Can you work these out from the drawing? Everything is in mm from the part's minimum corner. A direction names the side the tool comes from. Round coordinates to 2 decimals unless told otherwise and drop trailing zeros. Loops run counter-clockwise (first coordinate to the right, second up) from the corner with the lowest first, then second, coordinate; pieces in that order, holes last. Notation, with made-up numbers: (29, 57.25) -> (85, 57.25) arc R18 ccw to (85, 64.25) -> close; hole circle Ø6 at (69, -32). An arc over 180 degrees is marked (long way). One line per item, written item: value.
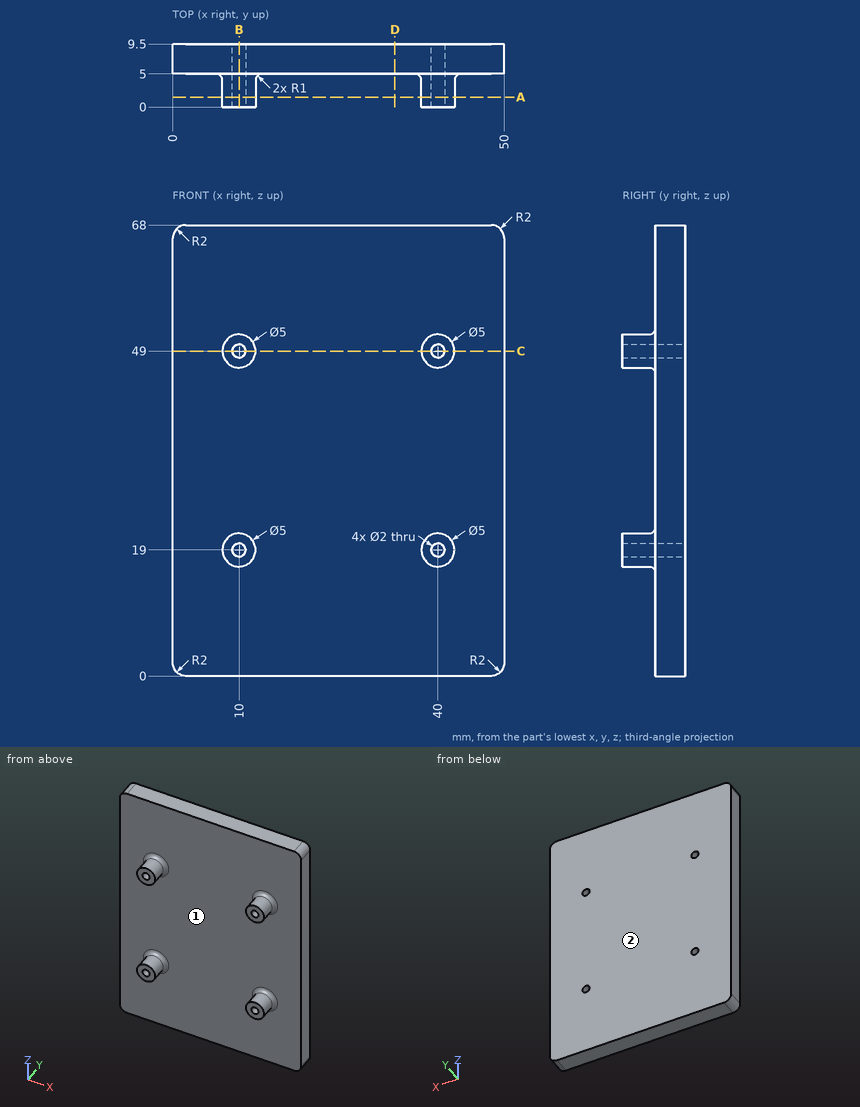
(1) On a 3-axis mill with a long thin cutter (end or side, diameter ignored), from which of +Z, -Z, +X, -X, +Y, -Y can I reach the whole of each face in a straight line? I mean the marked faces 1 and 2. Say none if no direction works.
Results below:
face 1: -Y
face 2: +Z, -Z, +X, -X, +Y
(2) Imagine slicing it at A-A on y = 1.5. Write out the boundary of the cut face in (x, z), then the cut area to 3 significant figures.
Results below:
outline: circle Ø5 at (10, 19); circle Ø5 at (10, 49); circle Ø5 at (40, 19); circle Ø5 at (40, 49); hole circle Ø2 at (10, 19); hole circle Ø2 at (10, 49); hole circle Ø2 at (40, 19); hole circle Ø2 at (40, 49)
area: 66.0 mm²
(3) Please list where these lines run through material, in increasing order: L1, parallel to Z at x = 40, y = 6.25; L2, parallel to X at y = 7.75, z = 49; L3, parallel to Y at x = 5, z = 54.
Results below:
L1: z = 0 to 18, 20 to 48, 50 to 68
L2: x = 0 to 9, 11 to 39, 41 to 50
L3: y = 5 to 9.5
(4) Imagine slicing it at D-D on x = 33.5. Write out the boundary of the cut face in (y, z), then the cut area to 3 significant figures.
Results below:
outline: (5, 0) -> (9.5, 0) -> (9.5, 68) -> (5, 68) -> close
area: 306 mm²
(5) Imagine slicing it at B-B on x = 10. Write out the boundary of the cut face in (y, z), then the cut area to 3 significant figures.
Results below:
outline: (0, 16.5) -> (4, 16.5) arc R1 cw to (5, 15.5) -> (5, 0) -> (9.5, 0) -> (9.5, 18) -> (0, 18) -> close; (0, 20) -> (9.5, 20) -> (9.5, 48) -> (0, 48) -> (0, 46.5) -> (4, 46.5) arc R1 cw to (5, 45.5) -> (5, 22.5) arc R1 cw to (4, 21.5) -> (0, 21.5) -> close; (0, 50) -> (9.5, 50) -> (9.5, 68) -> (5, 68) -> (5, 52.5) arc R1 cw to (4, 51.5) -> (0, 51.5) -> close
area: 319 mm²
(6) Imagine slicing it at C-C on z = 49. Write out the boundary of the cut face in (x, y).
Results below:
outline: (0, 5) -> (6.5, 5) arc R1 cw to (7.5, 4) -> (7.5, 0) -> (9, 0) -> (9, 9.5) -> (0, 9.5) -> close; (11, 0) -> (12.5, 0) -> (12.5, 4) arc R1 cw to (13.5, 5) -> (36.5, 5) arc R1 cw to (37.5, 4) -> (37.5, 0) -> (39, 0) -> (39, 9.5) -> (11, 9.5) -> close; (41, 0) -> (42.5, 0) -> (42.5, 4) arc R1 cw to (43.5, 5) -> (50, 5) -> (50, 9.5) -> (41, 9.5) -> close
(7) For pin 1 Ø3 at (x, z) = (10, 49) entering from +Y, with a flat end and sliding along its axis, tell me the tip position at first contact or that it passes through.
Results below:
pin 1: stops at y = 9.5
